```python
from build123d import *

# Parameters (mm, degrees)
BOSS_EXTRUDE1_DEPTH = 1


with BuildPart() as part:
    # Sketch1 → Boss-Extrude1 (new body)
    with BuildSketch(Plane.XY):
        Polygon((-180.819610652, -0.465116279), (-180.819610652, -15.465116279), (-175.819610652, -15.465116279), (-175.819610652, -0.465116279), (-170.819610652, -0.465116279), (-170.819610652, -15.465116279), (-165.819610652, -15.465116279), (-165.819610652, -0.465116279), (-160.819610652, -0.465116279), (-160.819610652, -15.465116279), (-155.819610652, -15.465116279), (-155.819610652, -0.465116279), (-150.819610652, -0.465116279), (-150.819610652, -15.465116279), (-145.819610652, -15.465116279), (-145.819610652, -0.465116279), (-140.819610652, -0.465116279), (-140.819610652, -15.465116279), (-135.819610652, -15.465116279), (-135.819610652, -0.465116279), (-130.819610652, -0.465116279), (-130.819610652, -15.465116279), (-125.819610652, -15.465116279), (-125.819610652, -0.465116279), (-120.819610652, -0.465116279), (-120.819610652, -15.465116279), (-115.819610652, -15.465116279), (-115.819610652, -0.465116279), (-110.819610652, -0.465116279), (-110.819610652, -15.465116279), (-105.819610652, -15.465116279), (-105.819610652, -0.465116279), (-100.819610652, -0.465116279), (-100.819610652, -15.465116279), (-95.819610652, -15.465116279), (-95.819610652, -0.465116279), (-90.819610652, -0.465116279), (-90.819610652, -15.465116279), (-85.819610652, -15.465116279), (-85.819610652, -0.465116279), (-80.819610652, -0.465116279), (-80.819610652, -15.465116279), (-75.819610652, -15.465116279), (-75.819610652, -0.465116279), (-70.819610652, -0.465116279), (-70.819610652, -15.465116279), (-65.819610652, -15.465116279), (-65.819610652, -0.465116279), (-60.819610652, -0.465116279), (-60.819610652, -15.465116279), (-55.819610652, -15.465116279), (-55.819610652, -0.465116279), (-50.819610652, -0.465116279), (-50.819610652, -15.465116279), (-45.819610652, -15.465116279), (-45.819610652, -0.465116279), (-40.819610652, -0.465116279), (-40.819610652, -15.465116279), (-35.819610652, -15.465116279), (-35.819610652, -0.465116279), (-30.819610652, -0.465116279), (-30.819610652, -15.465116279), (-25.819610652, -15.465116279), (-25.819610652, -0.465116279), (-20.819610652, -0.465116279), (-20.819610652, -15.465116279), (-15.819610652, -15.465116279), (-15.819610652, -0.465116279), (-10.819610652, -0.465116279), (-10.819610652, -15.465116279), (-5.819610652, -15.465116279), (-5.819610652, -0.465116279), (-0.819610652, -0.465116279), (-0.819610652, -15.465116279), (5.874690211, -15.465116279), (5.874690211, -0.465116279), (10.874690211, -0.465116279), (10.874690211, -15.465116279), (15.874690211, -15.465116279), (15.874690211, -0.465116279), (20.874690211, -0.465116279), (20.874690211, -15.465116279), (25.874690211, -15.465116279), (25.874690211, -0.465116279), (30.874690211, -0.465116279), (30.874690211, -15.465116279), (35.874690211, -15.465116279), (35.874690211, -0.465116279), (40.874690211, -0.465116279), (40.874690211, -15.465116279), (45.874690211, -15.465116279), (45.874690211, -0.465116279), (50.874690211, -0.465116279), (50.874690211, -15.465116279), (55.874690211, -15.465116279), (55.874690211, -0.465116279), (60.874690211, -0.465116279), (60.874690211, -15.465116279), (65.874690211, -15.465116279), (65.874690211, -0.465116279), (70.874690211, -0.465116279), (70.874690211, -15.465116279), (75.874690211, -15.465116279), (75.874690211, -0.465116279), (80.874690211, -0.465116279), (80.874690211, -15.465116279), (85.874690211, -15.465116279), (85.874690211, -0.465116279), (90.874690211, -0.465116279), (90.874690211, -15.465116279), (95.874690211, -15.465116279), (95.874690211, -0.465116279), (100.874690211, -0.465116279), (100.874690211, -15.465116279), (105.874690211, -15.465116279), (105.874690211, -0.465116279), (110.874690211, -0.465116279), (110.874690211, -15.465116279), (115.874690211, -15.465116279), (115.874690211, -0.465116279), (120.874690211, -0.465116279), (120.874690211, -15.465116279), (125.874690211, -15.465116279), (125.874690211, -0.465116279), (130.874690211, -0.465116279), (130.874690211, -15.465116279), (135.874690211, -15.465116279), (135.874690211, -0.465116279), (140.874690211, -0.465116279), (140.874690211, -15.465116279), (145.874690211, -15.465116279), (145.874690211, -0.465116279), (150.874690211, -0.465116279), (150.874690211, -15.465116279), (155.874690211, -15.465116279), (155.874690211, -0.465116279), (160.874690211, -0.465116279), (160.874690211, -15.465116279), (165.874690211, -15.465116279), (165.874690211, -0.465116279), (170.874690211, -0.465116279), (170.874690211, -15.465116279), (177.52753978, -15.465116279), (177.52753978, 19.534883721), (-202.47246022, 19.534883721), (-202.47246022, -15.465116279), (-195.819610652, -15.465116279), (-195.819610652, -0.465116279), (-190.819610652, -0.465116279), (-190.819610652, -15.465116279), (-185.819610652, -15.465116279), (-185.819610652, -0.465116279), align=None)
    extrude(amount=BOSS_EXTRUDE1_DEPTH)


solid = part.part
```
Work out the finished part from the listing and answer in its coordinate system (mm). Give positions to 0.01 mm unless a question says otherwise; leave off trailing zeros.
(1) A straight line is drawn through the part: line 1 (Y direction, x = -155, z = 0.95). Find the intervals that lie inside material, in ascending order.
Final values:
line 1: y = -0.47 to 19.53
(2) The part is cut by section A-A on y = -5. Count the separate pieces of the cut face and the enclosed holes in it, plus the area to 3 significant figures.
Final values:
separate pieces: 38
enclosed holes: 0
area: 195 mm2
(3) A flat-ended cylindrical pin translates along its axis: pin 1 Ø3 at (x, y) = (-10, -12) entering from -Z. Find the tip coordinate at first contact, or state that the pin passes through.
Final values:
pin 1: stops at z = 0
